Source: CAD feature listing. Evaluate the final solid. Frame: model axes, mm. A direction names the side the tool comes from. Give positions to 0.01 mm unless a question says otherwise; leave off trailing zeros. Order: outer loops, then holes, each group sorted by start corner. A loop starts at its lowest first (then second) coordinate and runs counter-clockwise, first axis right, second up. Notation, with made-up numbers: (60.25, 75) -> (82.25, 75) arc R34 cw to (82.25, 110) -> close; hole circle Ø8 at (-0.5, 22). An arc over 180 degrees is marked (long way). Answer in a Markdown table with one row per item.
Autodesk Fusion 360 part; units mm, degrees
sketch "mriya-niceview-holder" plane through (0, 0, 0) normal (0, 0, 1) x (1, 0, 0)
  line L0 (-20.8, 9.9) -> (-9.8, 9.9)
  line L1 (-9.8, 9.9) -> (-9.8, 36.9)
  line L2 (-22.3, 3.9) -> (-22.3, 36.9)
  line L3 (-20.8, 9.9) -> (-20.8, 36.9)
  line L4 (-8.3, 36.9) -> (-8.3, 3.9)
  line L5 (-22.3, 36.9) -> (-19.8, 36.9)
  line L6 (-22.3, 3.9) -> (-8.3, 3.9)
  arc A0 (-19.8, 34.9) -> (-18.8, 33.9) centre (-18.8, 34.9) ccw
  line L7 (-10.8, 36.9) -> (-8.3, 36.9)
  arc A1 (-11.8, 33.9) -> (-10.8, 34.9) centre (-11.8, 34.9) ccw
  line L8 (-10.8, 34.9) -> (-10.8, 36.9)
  line L9 (-18.8, 33.9) -> (-11.8, 33.9)
  line L10 (-19.8, 34.9) -> (-19.8, 36.9)
extrude "Extrude1" add sketch "mriya-niceview-holder" along normal blind 2 contours L0 L1 L2 L3 L4 L5 L6 L7
extrude "Extrude2" add sketch "mriya-niceview-holder" along normal blind 0.8 contours L0 L1 L3 L5 A0 L7 A1 L8 L9 L10
chamfer "Chamfer4" distance 0.6 angle 45 2 edges at (-22.3, 20.4, 0) (-8.3, 20.4, 0)
fillet "Fillet1" radius 1 4 edges at (-8.3, 3.9, 1) (-22.3, 3.9, 1) (-8.3, 36.9, 1) (-22.3, 36.9, 1)
fillet "Fillet2" radius 0.5 2 edges at (-10.8, 36.9, 0.4) (-19.8, 36.9, 0.4)
fillet "Fillet3" radius 1 2 edges at (-20.8, 9.9, 1.4) (-9.8, 9.9, 1.4)
(1) Section query D-D (x = -11.25). Return the cut outline in (y, z), plus the area to 3 significant figures.
A:
| item | result |
|---|---|
| outline | (3.9, 0) -> (34.06, 0) -> (34.06, 0.8) -> (9.9, 0.8) -> (9.9, 2) -> (3.9, 2) -> close |
| area | 31.3 mm^2 |
(2) Section query B-B (x = -16). Return the cut outline in (y, z).
A:
| item | result |
|---|---|
| outline | (3.9, 0) -> (33.9, 0) -> (33.9, 0.8) -> (9.9, 0.8) -> (9.9, 2) -> (3.9, 2) -> close |
(3) Ray query, probe 1 along X at (y, z) = (24, 0.9); probe 2 along X at (y, z) = (35.5, 0.65); probe 3 along Y at (x, z) = (-14.25, 1.55). Return the intervals inside material, ascending.
A:
| item | result |
|---|---|
| probe 1 | x = -22.3 to -20.8, -9.8 to -8.3 |
| probe 2 | x = -22.3 to -19.8, -10.8 to -8.3 |
| probe 3 | y = 3.9 to 9.9 |
(4) Section query C-C (y = 21). Return the cut outline in (x, z), plus the area to 3 significant figures.
A:
| item | result |
|---|---|
| outline | (-22.3, 0.6) -> (-21.7, 0) -> (-8.9, 0) -> (-8.3, 0.6) -> (-8.3, 2) -> (-9.8, 2) -> (-9.8, 0.8) -> (-20.8, 0.8) -> (-20.8, 2) -> (-22.3, 2) -> close |
| area | 14.4 mm^2 |
(5) Access query for faces 1 (the flat face through (-9.8, 24, 1)), 2 (the flat face through (-22.3, 20, 1)), 3 (the cylindrical face through (-19.499, 34.185, 0.394)). Directions: +Z, -Z, +X, -X, +Y, -Y. A direction counts if a zero-diameter tool reaches every point of the face in a straight line with its end or side. Return the directions, or none.
A:
| item | result |
|---|---|
| face 1 | +Z, +Y |
| face 2 | +Z, -Z, -X, +Y, -Y |
| face 3 | +Z, -Z, +Y |
(6) Section query A-A (z = 1.6). Return the cut outline in (x, y), plus the area to 3 significant figures.
A:
| item | result |
|---|---|
| outline | (-22.3, 4.9) arc R1 ccw to (-21.3, 3.9) -> (-9.3, 3.9) arc R1 ccw to (-8.3, 4.9) -> (-8.3, 35.9) arc R1 ccw to (-9.3, 36.9) -> (-9.8, 36.9) -> (-9.8, 10.9) arc R1 cw to (-10.8, 9.9) -> (-19.8, 9.9) arc R1 cw to (-20.8, 10.9) -> (-20.8, 36.9) -> (-21.3, 36.9) arc R1 ccw to (-22.3, 35.9) -> close |
| area | 165 mm^2 |
(7) First-contact query: pin 1 Ø0.6 at (x, z) = (-17, 1) entering from +Y; pin 2 Ø3.5 at (x, y) = (-15.5, 29) entering from +Z. Flat tips, straight axial feed; report the tip coordinate or a pass-through.
A:
| item | result |
|---|---|
| pin 1 | stops at y = 33.9 |
| pin 2 | stops at z = 0.8 |
